Could you check a few things on this model? Use its own coordinates, in mm. Face numbers are marked on the shaded views. A direction names the side the tool comes from. Give positions to 0.01 mm unless a question says otherwise; leave off trailing zeros. Order: outer loops, then holes, each group sorted by start corner. A loop starts at its lowest first (then second) coordinate and runs counter-clockwise, first axis right, second up. Notation, with made-up numbers: M 77,36.25 L 134,36.25 A35 ccw 134,75.25 Z; hole C 68.25,14 d8. An arc over 180 degrees is marked long. Use a Markdown table: item, result. Add a question column.
```python
from build123d import *

# Parameters (mm, degrees)
BOSS_EXTRUDE1_OUTLINE_W                             = 55
BOSS_EXTRUDE1_OUTLINE_H                             = 40
BOSS_EXTRUDE1_DEPTH                                 = 10
SKETCH5_W                                           = 40
SKETCH5_H                                           = 14
BOSS_EXTRUDE2_DEPTH                                 = 40
CUT_EXTRUDE3_DEPTH                                  = 74
SKETCH7_W                                           = 40
SKETCH7_H                                           = 6
BOSS_EXTRUDE3_DEPTH                                 = 14
SKETCH11_W                                          = 40
SKETCH11_H                                          = 28
BOSS_EXTRUDE5_DEPTH                                 = 4
SKETCH12_W                                          = 40
SKETCH12_H                                          = 24
SKETCH12_H_2                                        = 20
BOSS_EXTRUDE6_DEPTH                                 = 3
FILLET1_R                                           = 5
SKETCH23_R                                          = 3
CUT_EXTRUDE11_DEPTH                                 = 10
SKETCH26_R                                          = 4.325
CUT_EXTRUDE12_DEPTH                                 = 4.1
CUT_EXTRUDE13_DEPTH                                 = 1.5
CBORE_FOR_M4_HEX_SOCKET_HEAD_CAP_SCREW1_D           = 4.5
CBORE_FOR_M4_HEX_SOCKET_HEAD_CAP_SCREW1_CBORE_D     = 8
CBORE_FOR_M4_HEX_SOCKET_HEAD_CAP_SCREW1_CBORE_DEPTH = 4.4


# Read off the part's stored shape, not the designer's step: Boss-Extrude1
with BuildPart() as part:
    # Boss-Extrude1 outline → Boss-Extrude1 (new body)
    with BuildSketch(Plane.XY):
        with Locations((7.5, 0)):
            Rectangle(BOSS_EXTRUDE1_OUTLINE_W, BOSS_EXTRUDE1_OUTLINE_H)
    extrude(amount=BOSS_EXTRUDE1_DEPTH)

    # Sketch5 → Boss-Extrude2 (add, symmetric)
    with BuildSketch(Plane(origin=(0, 0, 0), x_dir=(1, 0, 0), z_dir=(0, 1, 0))):
        with Locations((15, -10)):
            Rectangle(SKETCH5_W, SKETCH5_H)
    extrude(amount=BOSS_EXTRUDE2_DEPTH, both=True)

    # Sketch6 → Cut-Extrude3 (cut)
    with BuildSketch(Plane(origin=(0, 34, 0), x_dir=(1, 0, 0), z_dir=(0, 1, 0))):
        Polygon((-1.5, -8.5), (31.5, -8.5), (27.169033679, -17), (2.830966321, -17), align=None)
    extrude(amount=-CUT_EXTRUDE3_DEPTH, mode=Mode.SUBTRACT)

    # Sketch7 → Boss-Extrude3 (add)
    with BuildSketch(Plane.XY.offset(17)):
        with Locations((15, 37)):
            Rectangle(SKETCH7_W, SKETCH7_H)
    extrude(amount=BOSS_EXTRUDE3_DEPTH)

    # Sketch11 → Boss-Extrude5 (add)
    with BuildSketch(Plane(origin=(0, 40, 0), x_dir=(1, 0, 0), z_dir=(0, 1, 0))):
        with Locations((15, -17)):
            Rectangle(SKETCH11_W, SKETCH11_H)
    extrude(amount=BOSS_EXTRUDE5_DEPTH)

    # Sketch12 → Boss-Extrude6 (add)
    with BuildSketch(Plane(origin=(0, 0, 3), x_dir=(-1, 0, 0), z_dir=(0, 0, -1))):
        with Locations((-15, 32)):
            Rectangle(SKETCH12_W, SKETCH12_H)
        with Locations((-15, -30)):
            Rectangle(SKETCH12_W, SKETCH12_H_2)
    extrude(amount=BOSS_EXTRUDE6_DEPTH)

    # Fillet1
    fillet1_edges = [part.edges().sort_by_distance(p)[0] for p in [
        (-5, -20, 5),
        (-5, 20, 5),
        (-20, 20, 5),
        (-20, -20, 5),
    ]]
    fillet(fillet1_edges, radius=FILLET1_R)

    # Sketch23 → Cut-Extrude11 (cut)
    with BuildSketch(Plane(origin=(0, 44, 0), x_dir=(1, 0, 0), z_dir=(0, 1, 0))):
        with Locations(Location((0, -5, 0), (0, 0, 180))):
            Circle(SKETCH23_R)
        with Locations(Location((30, -5, 0), (0, 0, 180))):
            Circle(SKETCH23_R)
        with Locations(Location((30, -26, 0), (0, 0, 180))):
            Circle(SKETCH23_R)
        with Locations(Location((0, -26, 0), (0, 0, 180))):
            Circle(SKETCH23_R)
    extrude(amount=-CUT_EXTRUDE11_DEPTH, mode=Mode.SUBTRACT)

    # Sketch25 → Cut-Revolve1 (revolve, cut)
    with BuildSketch(Plane.XY.offset(18.5), mode=Mode.PRIVATE) as cut_revolve1_sk:
        Polygon((15, 44), (15, 38.1), (19.325, 38.1), (23.725, 42.5), (23.725, 44), align=None)
    revolve(cut_revolve1_sk.sketch.rotate(Axis((15, 44, 18.5), (0, -1, 0)), 90), axis=Axis((15, 44, 18.5), (0, -1, 0)), mode=Mode.SUBTRACT)

    # Sketch26 → Cut-Extrude12 (cut)
    with BuildSketch(Plane(origin=(0, 38.1, 0), x_dir=(1, 0, 0), z_dir=(0, 1, 0))):
        with Locations(Location((15, -18.5, 0), (0, 0, 270))):
            Circle(SKETCH26_R)
    extrude(amount=-CUT_EXTRUDE12_DEPTH, mode=Mode.SUBTRACT)

    # Sketch28 → Cut-Extrude13 (cut)
    with BuildSketch(Plane.XY.offset(10)):
        with BuildLine():
            Line((-15, -20), (-10, -20))
            ThreePointArc((-10, -20), (-6.464466094, -21.464466094), (-5, -25))
            Line((-5, -25), (-5, 25))
            ThreePointArc((-5, 25), (-6.464466094, 21.464466094), (-10, 20))
            Line((-10, 20), (-15, 20))
            ThreePointArc((-15, 20), (-18.535533906, 18.535533906), (-20, 15))
            Line((-20, 15), (-20, -15))
            ThreePointArc((-20, -15), (-18.535533906, -18.535533906), (-15, -20))
        make_face()
    extrude(amount=-CUT_EXTRUDE13_DEPTH, mode=Mode.SUBTRACT)

    # CBORE for M4 Hex Socket Head Cap Screw1 (through all)
    with Locations(Plane.XY.offset(8.5)):
        with Locations((-12, 12), (12, 12), (12, -12), (-12, -12)):
            CounterBoreHole(CBORE_FOR_M4_HEX_SOCKET_HEAD_CAP_SCREW1_D / 2, CBORE_FOR_M4_HEX_SOCKET_HEAD_CAP_SCREW1_CBORE_D / 2, CBORE_FOR_M4_HEX_SOCKET_HEAD_CAP_SCREW1_CBORE_DEPTH)


solid = part.part
```
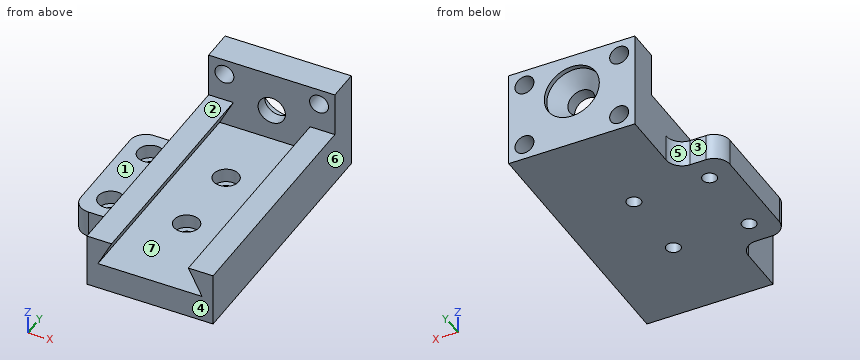
1) For pin 1 (5.5 mm diameter, centred on x = -12, z = 3.5, fed in from +Y); pin 2 (2.5 mm diameter, centred on x = 10.5, y = 10, fed in from +Z); pin 3 (6.5 mm diameter, centred on x = -11, y = -11.5, fed in from +Z); pin 4 (3 mm diameter, centred on y = -15, z = 19, fed in from -X), each with a flat end and sliding along its axis, tell me the tip position at first contact or that it passes through.
2) Suppose I cut it at C-C on x = -12. Please give me the cut outline in (y, z), and give its area (3 significant figures).
3) Suppose I cut it at B-B on y = 12. Please give me the cut outline in (x, z).
4) Please list where these lines run through material, in increasing order: line 1 (Z direction, x = 30, y = 40.25); line 2 (Y direction, x = 12, z = 7.45); line 3 (Y direction, x = 12, z = 1.3). Write a range as from..to.
5) We'd pull the mould along X, two halves only. Please class the marked faces 4, 5, 6 and 7: pulls with the +X half, pulls with the -X half, needs draft (parallel to the pull), parting line crosses it, or undercut.
6) Suppose I cut it at A-A on z = 18.5. Please give me the cut outline in (x, y) (3 decimals).
7) Suppose I cut it at D-D on z = 5. Please give me the cut outline in (x, y), and give its area (3 significant figures).
8) For the marked faces 1, 2 and 3, which set-ups out of +Z, -Z, +X, -X, +Y, -Y let a thin tool reach every point of the face, with its end or its side?
Values found:
| question | item | result |
|---|---|---|
| 1 | pin 1 | stops at y = 20.06 |
| 1 | pin 2 | stops at z = 4.1 |
| 1 | pin 3 | stops at z = 8.5 |
| 1 | pin 4 | passes through |
| 2 | outline | M -20,0 L -14.25,0 L -14.25,4.1 L -16,4.1 L -16,8.5 L -20,8.5 Z; M -9.75,0 L 9.75,0 L 9.75,4.1 L 8,4.1 L 8,8.5 L -8,8.5 L -8,4.1 L -9.75,4.1 Z; M 14.25,0 L 20,0 L 20,8.5 L 16,8.5 L 16,4.1 L 14.25,4.1 Z |
| 2 | area | 233 mm^2 |
| 3 | outline | M -20,0 L -14.25,0 L -14.25,4.1 L -16,4.1 L -16,8.5 L -20,8.5 Z; M -9.75,0 L 9.75,0 L 9.75,4.1 L 8,4.1 L 8,8.5 L -1.5,8.5 L 2.83,17 L -5,17 L -5,8.5 L -8,8.5 L -8,4.1 L -9.75,4.1 Z; M 14.25,0 L 35,0 L 35,17 L 27.17,17 L 31.5,8.5 L 16,8.5 L 16,4.1 L 14.25,4.1 Z |
| 4 | line 1 | z = 0..2, 8..23, 29..31 |
| 4 | line 2 | y = -40..-16, -8..8, 16..44 |
| 4 | line 3 | y = -40..-14.25, -9.75..9.75, 14.25..44 |
| 5 | face 4 | needs draft |
| 5 | face 5 | pulls with the -X half |
| 5 | face 6 | pulls with the +X half |
| 5 | face 7 | undercut |
| 6 | outline | M -5,34 L 10.675,34 L 10.675,38.1 L 6.275,42.5 L 6.275,44 L -5,44 Z; M 19.325,34 L 35,34 L 35,44 L 23.725,44 L 23.725,42.5 L 19.325,38.1 Z |
| 7 | outline | M -20,-15 A5 ccw -15,-20 L -10,-20 A5 cw -5,-25 L -5,-40 L 35,-40 L 35,44 L 33,44 L 33,34 L 27,34 L 27,44 L 3,44 L 3,34 L -3,34 L -3,44 L -5,44 L -5,25 A5 cw -10,20 L -15,20 A5 ccw -20,15 Z; hole C -12,-12 d8; hole C -12,12 d8; hole C 12,-12 d8; hole C 12,12 d8 |
| 7 | area | 3,640 mm^2 |
| 8 | face 1 | +Z, -X, +Y, -Y |
| 8 | face 2 | +Z, +X, -X, -Y |
| 8 | face 3 | +Z, -Z, -X, +Y |
